For this review, take the finished solid that the model builds, in its own axes (mm). A direction names the side the tool comes from. Coordinates: 2 decimals unless noted, no trailing zeros. Write each loop counter-clockwise with the first axis right and the second up, starting at its lowest first coordinate (ties: lowest second). Pieces come first, ordered by that corner, then holes. Notation, with made-up numbers: (83.25, 80) -> (118.25, 80) arc R35 cw to (118.25, 112) -> close; hole circle Ø1 at (71.25, 13). An arc over 180 degrees is marked (long way). Put each result on its own line as item: value. Start each with the question number.
Item 1: Consider section B-B on x = -6. Give the boundary of the cut face in (y, z), and give its area (3 significant figures).
Item 2: The part is to be moulded in two halves that separate along Y. For faces 1 (the cylindrical face through (-1.465, 57.154, 80.507)), 2 (the cylindrical face through (18.9, 29.7, -29.5)), 3 (the flat face through (-10, 8, 25)), 4 (the flat face through (0, 30, -30)), say which applies: +Y half, -Y half, draft (parallel to the pull), parting line (faces both ways), or undercut.
Item 3: To check wall thickness, follow L1, parallel to Y at x = 0, z = 80.4; L2, parallel to X at y = 23, z = 5.5; L3, parallel to Z at x = 26.5, y = 20.5. State the ranges of each line that lie inside material, in increasing order.
Item 4: Insertion check: P1, Ø2.5, axis at x = -16, z = 32.5, coming from the +Y side; P2, Ø1.6, axis at x = -10.5, z = 24.5, coming from the +Y side; P3, Ø18.5, axis at x = 0, y = 46, coming from the +Z side. Each pin has a flat end and moves straight along its axis. Give the tip position at first contact, or say it passes through.
Item 5: Consider section D-D on z = -16.5. Give the boundary of the cut face in (x, y), and give its area (3 significant figures).
Item 6: Consider section C-C on y = 10.5. Give the boundary of the cut face in (x, z), and give its area (3 significant figures).
Item 7: For faces 5 (the flat face through (5.07, 0.51, -8.62)), 6 (the cylindrical face through (-16.019, 3.465, 79.526)), 7 (the flat face through (-32, 23, 26)), list the 3-axis set-ups (+Z, -Z, +X, -X, +Y, -Y) from which the entire face can be reached by the end or side of a thin tool; tool diameter is ignored.
Item 8: Consider section A-A on z = 52.5. Give the boundary of the cut face in (x, y).
```python
from build123d import *

# Parameters (mm, degrees)
IZIM1_W                     = 60
IZIM1_H                     = 60
Y_KSEKLIK_EKSTR_ZYON1_DEPTH = 1
IZIM2_R                     = 1.6
Y_KSEKLIK_EKSTR_ZYON2_DEPTH = 7
IZIM3_W                     = 60
IZIM3_H                     = 1
Y_KSEKLIK_EKSTR_ZYON3_DEPTH = 2
IZIM4_W                     = 39
IZIM4_H                     = 1
Y_KSEKLIK_EKSTR_ZYON4_DEPTH = 51
IZIM5_R                     = 1.6
Y_KSEKLIK_EKSTR_ZYON5_DEPTH = 5
IZIM6_W                     = 51
IZIM6_H                     = 1
Y_KSEKLIK_EKSTR_ZYON6_DEPTH = 12.5
IZIM7_W                     = 51
IZIM7_H                     = 1
Y_KSEKLIK_EKSTR_ZYON7_DEPTH = 12.5
KES_EKSTR_ZYON1_DEPTH       = 88.372764635
IZIM9_W                     = 64
IZIM9_H                     = 111
IZIM9_W_2                   = 62
IZIM9_H_2                   = 109
Y_KSEKLIK_EKSTR_ZYON8_DEPTH = 60
KES_EKSTR_ZYON2_REACH       = 132.637
IZIM10_R                    = 11.25
IZIM10_W                    = 32
IZIM10_H                    = 12
KES_EKSTR_ZYON3_REACH       = 121.908
IZIM11_R                    = 11.25
KES_EKSTR_ZYON4_REACH       = 132.637
IZIM12_R                    = 8
IZIM12_R_2                  = 2.55
KES_EKSTR_ZYON5_REACH       = 132.637
IZIM14_W                    = 9
IZIM14_H                    = 11.4


with BuildPart() as part:
    # Çizim1 → Yükseklik-Ekstrüzyon1 (new body)
    with BuildSketch(Plane(origin=(0, 0, 0), x_dir=(1, 0, 0), z_dir=(0, 1, 0))):
        Rectangle(IZIM1_W, IZIM1_H)
    extrude(amount=Y_KSEKLIK_EKSTR_ZYON1_DEPTH)

    # Çizim2 → Yükseklik-Ekstrüzyon2 (add)
    with BuildSketch(Plane(origin=(0, 1, 0), x_dir=(1, 0, 0), z_dir=(0, 1, 0))):
        with Locations(Location((-10, -25, 0), (0, 0, 270))):
            Circle(IZIM2_R)
        with Locations(Location((15, -25, 0), (0, 0, 270))):
            Circle(IZIM2_R)
        with Locations(Location((-10, 27, 0), (0, 0, 270))):
            Circle(IZIM2_R)
        with Locations(Location((15, 27, 0), (0, 0, 270))):
            Circle(IZIM2_R)
    extrude(amount=Y_KSEKLIK_EKSTR_ZYON2_DEPTH)

    # Çizim3 → Yükseklik-Ekstrüzyon3 (add)
    with BuildSketch(Plane(origin=(30, 0, 0), x_dir=(0, 0, -1), z_dir=(1, 0, 0))):
        with Locations((0, 0.5)):
            Rectangle(IZIM3_W, IZIM3_H)
    y_kseklik_ekstr_zyon3 = extrude(amount=Y_KSEKLIK_EKSTR_ZYON3_DEPTH)

    # Aynalama1: Yükseklik-Ekstrüzyon3 across plane
    add(y_kseklik_ekstr_zyon3.mirror(Plane(origin=(0, 0, 0), x_dir=(0, 0, 1), z_dir=(1, 0, 0))))

    # Çizim4 → Yükseklik-Ekstrüzyon4 (add)
    with BuildSketch(Plane.XY.offset(30)):
        with Locations((0, 0.5)):
            Rectangle(IZIM4_W, IZIM4_H)
    extrude(amount=Y_KSEKLIK_EKSTR_ZYON4_DEPTH)

    # Çizim5 → Yükseklik-Ekstrüzyon5 (add)
    with BuildSketch(Plane(origin=(0, 1, 0), x_dir=(1, 0, 0), z_dir=(0, 1, 0))):
        with Locations(Location((-16.5, -32, 0), (0, 0, 270))):
            Circle(IZIM5_R)
        with Locations(Location((16.5, -32, 0), (0, 0, 90))):
            Circle(IZIM5_R)
        with Locations(Location((-16.5, -78, 0), (0, 0, 270))):
            Circle(IZIM5_R)
        with Locations(Location((16.5, -78, 0), (0, 0, 90))):
            Circle(IZIM5_R)
    extrude(amount=Y_KSEKLIK_EKSTR_ZYON5_DEPTH)

    # Çizim6 → Yükseklik-Ekstrüzyon6 (add)
    with BuildSketch(Plane(origin=(19.5, 0, 0), x_dir=(0, 0, -1), z_dir=(1, 0, 0))):
        with Locations((-55.5, 0.5)):
            Rectangle(IZIM6_W, IZIM6_H)
    extrude(amount=Y_KSEKLIK_EKSTR_ZYON6_DEPTH)

    # Çizim7 → Yükseklik-Ekstrüzyon7 (add)
    with BuildSketch(Plane.ZY.offset(19.5)):
        with Locations((55.5, 0.5)):
            Rectangle(IZIM7_W, IZIM7_H)
    extrude(amount=Y_KSEKLIK_EKSTR_ZYON7_DEPTH)

    # Çizim8 → Kes-Ekstrüzyon1 (cut, through all)
    with BuildSketch(Plane(origin=(0, 1, 0), x_dir=(1, 0, 0), z_dir=(0, 1, 0))):
        Polygon((-10, -5.773502692), (0, -11.547005384), (10, -5.773502692), (10, 5.773502692), (0, 11.547005384), (-10, 5.773502692), align=None)
        Polygon((-10, -60.226497308), (0, -66), (10, -60.226497308), (10, -48.679491924), (0, -42.905989232), (-10, -48.679491924), align=None)
    extrude(amount=-KES_EKSTR_ZYON1_DEPTH, mode=Mode.SUBTRACT)

    # Çizim9 → Yükseklik-Ekstrüzyon8 (add)
    with BuildSketch(Plane(origin=(0, 1, 0), x_dir=(1, 0, 0), z_dir=(0, 1, 0))):
        with Locations((0, -25.5)):
            Rectangle(IZIM9_W, IZIM9_H)
        with Locations((0, -25.5)):
            Rectangle(IZIM9_W_2, IZIM9_H_2, mode=Mode.SUBTRACT)
    extrude(amount=Y_KSEKLIK_EKSTR_ZYON8_DEPTH)

    # Çizim10 → Kes-Ekstrüzyon2 (cut, up to next)
    with BuildSketch(Plane.XY.offset(81), mode=Mode.PRIVATE) as kes_ekstr_zyon2_sk1:
        with Locations((0, 46)):
            Circle(IZIM10_R)
    kes_ekstr_zyon2_tool1 = extrude(kes_ekstr_zyon2_sk1.sketch, amount=-KES_EKSTR_ZYON2_REACH, mode=Mode.PRIVATE) & part.part
    # Çizim10 → Kes-Ekstrüzyon2 (cut, up to next)
    with BuildSketch(Plane.XY.offset(81), mode=Mode.PRIVATE) as kes_ekstr_zyon2_sk2:
        with Locations((0, 23)):
            Rectangle(IZIM10_W, IZIM10_H)
    kes_ekstr_zyon2_tool2 = extrude(kes_ekstr_zyon2_sk2.sketch, amount=-KES_EKSTR_ZYON2_REACH, mode=Mode.PRIVATE) & part.part
    add(kes_ekstr_zyon2_tool1.solids().sort_by_distance((0, 46, 81))[0], mode=Mode.SUBTRACT)
    add(kes_ekstr_zyon2_tool2.solids().sort_by_distance((0, 23, 81))[0], mode=Mode.SUBTRACT)

    # Çizim11 → Kes-Ekstrüzyon3 (cut, up to next)
    with BuildSketch(Plane.ZY.offset(32), mode=Mode.PRIVATE) as kes_ekstr_zyon3_sk1:
        with Locations((25.5, 41)):
            Circle(IZIM11_R)
    kes_ekstr_zyon3_tool1 = extrude(kes_ekstr_zyon3_sk1.sketch, amount=-KES_EKSTR_ZYON3_REACH, mode=Mode.PRIVATE) & part.part
    add(kes_ekstr_zyon3_tool1.solids().sort_by_distance((-32, 41, 25.5))[0], mode=Mode.SUBTRACT)

    # Çizim12 → Kes-Ekstrüzyon4 (cut, up to next)
    with BuildSketch(Plane(origin=(0, 0, -30), x_dir=(-1, 0, 0), z_dir=(0, 0, -1)), mode=Mode.PRIVATE) as kes_ekstr_zyon4_sk1:
        with Locations((0, 46)):
            Circle(IZIM12_R)
    kes_ekstr_zyon4_tool1 = extrude(kes_ekstr_zyon4_sk1.sketch, amount=-KES_EKSTR_ZYON4_REACH, mode=Mode.PRIVATE) & part.part
    # Çizim12 → Kes-Ekstrüzyon4 (cut, up to next)
    with BuildSketch(Plane(origin=(0, 0, -30), x_dir=(-1, 0, 0), z_dir=(0, 0, -1)), mode=Mode.PRIVATE) as kes_ekstr_zyon4_sk2:
        with Locations((-17, 28)):
            Circle(IZIM12_R_2)
    kes_ekstr_zyon4_tool2 = extrude(kes_ekstr_zyon4_sk2.sketch, amount=-KES_EKSTR_ZYON4_REACH, mode=Mode.PRIVATE) & part.part
    # Çizim12 → Kes-Ekstrüzyon4 (cut, up to next)
    with BuildSketch(Plane(origin=(0, 0, -30), x_dir=(-1, 0, 0), z_dir=(0, 0, -1)), mode=Mode.PRIVATE) as kes_ekstr_zyon4_sk3:
        with BuildLine():
            Line((16.5, 30.05), (17.5, 30.05))
            ThreePointArc((17.5, 30.05), (19.55, 28), (17.5, 25.95))
            Line((17.5, 25.95), (16.5, 25.95))
            ThreePointArc((16.5, 25.95), (14.45, 28), (16.5, 30.05))
        make_face()
    kes_ekstr_zyon4_tool3 = extrude(kes_ekstr_zyon4_sk3.sketch, amount=-KES_EKSTR_ZYON4_REACH, mode=Mode.PRIVATE) & part.part
    add(kes_ekstr_zyon4_tool1.solids().sort_by_distance((0, 46, -30))[0], mode=Mode.SUBTRACT)
    add(kes_ekstr_zyon4_tool2.solids().sort_by_distance((17, 28, -30))[0], mode=Mode.SUBTRACT)
    add(kes_ekstr_zyon4_tool3.solids().sort_by_distance((-17, 28, -30))[0], mode=Mode.SUBTRACT)

    # Çizim14 → Kes-Ekstrüzyon5 (cut, up to next)
    with BuildSketch(Plane(origin=(0, 0, -30), x_dir=(-1, 0, 0), z_dir=(0, 0, -1)), mode=Mode.PRIVATE) as kes_ekstr_zyon5_sk1:
        with Locations((-26.5, 10.7)):
            Rectangle(IZIM14_W, IZIM14_H)
    kes_ekstr_zyon5_tool1 = extrude(kes_ekstr_zyon5_sk1.sketch, amount=-KES_EKSTR_ZYON5_REACH, mode=Mode.PRIVATE) & part.part
    # Çizim14 → Kes-Ekstrüzyon5 (cut, up to next)
    with BuildSketch(Plane(origin=(0, 0, -30), x_dir=(-1, 0, 0), z_dir=(0, 0, -1)), mode=Mode.PRIVATE) as kes_ekstr_zyon5_sk2:
        with BuildLine():
            Line((-2.25, 19.5), (2.25, 19.5))
            ThreePointArc((2.25, 19.5), (4.25, 17.5), (2.25, 15.5))
            Line((2.25, 15.5), (-2.25, 15.5))
            ThreePointArc((-2.25, 15.5), (-4.25, 17.5), (-2.25, 19.5))
        make_face()
    kes_ekstr_zyon5_tool2 = extrude(kes_ekstr_zyon5_sk2.sketch, amount=-KES_EKSTR_ZYON5_REACH, mode=Mode.PRIVATE) & part.part
    add(kes_ekstr_zyon5_tool1.solids().sort_by_distance((26.5, 10.7, -30))[0], mode=Mode.SUBTRACT)
    add(kes_ekstr_zyon5_tool2.solids().sort_by_distance((0, 17.5, -30))[0], mode=Mode.SUBTRACT)


solid = part.part
```
Return value:
1. outline: (0, -30) -> (40.71, -30) -> (40.71, -29) -> (1, -29) -> (1, -8.08) -> (0, -8.08) -> close; (0, 8.08) -> (1, 8.08) -> (1, 46.37) -> (0, 46.37) -> close; (0, 62.54) -> (1, 62.54) -> (1, 80) -> (17, 80) -> (17, 81) -> (0, 81) -> close; (29, 80) -> (36.48, 80) -> (36.48, 81) -> (29, 81) -> close; (51.29, -30) -> (61, -30) -> (61, -29) -> (51.29, -29) -> close; (55.52, 80) -> (61, 80) -> (61, 81) -> (55.52, 81) -> close
1. area: 157 mm^2
2. face 1: undercut
2. face 2: undercut
2. face 3: +Y half
2. face 4: draft
3. L1: 0 to 17, 29 to 34.75, 57.25 to 61
3. L2: -32 to -31, 31 to 32
3. L3: -30 to -29, 80 to 81
4. P1: y = 6
4. P2: y = 8
4. P3: z = -29
5. outline: (-32, 0) -> (32, 0) -> (32, 61) -> (31, 61) -> (31, 1) -> (-31, 1) -> (-31, 61) -> (-32, 61) -> close
5. area: 184 mm^2
6. outline: (-32, -30) -> (22, -30) -> (22, -29) -> (-31, -29) -> (-31, 80) -> (31, 80) -> (31, -30) -> (32, -30) -> (32, 81) -> (-32, 81) -> close
6. area: 337 mm^2
7. face 5: +Y, -Y
7. face 6: +Y
7. face 7: +Z, -Z, -X, +Y, -Y
8. outline: (-32, 0) -> (-10, 0) -> (-10, 1) -> (-31, 1) -> (-31, 61) -> (-32, 61) -> close; (10, 0) -> (32, 0) -> (32, 61) -> (31, 61) -> (31, 1) -> (10, 1) -> close
